from build123d import *

# Parameters (mm, degrees)
F1_DEPTH      = 2.5
F2_SIZE       = 4
F3_SIZE       = 1.99999
F4_R          = 2.49999
F5_R          = 1
F6_DEPTH      = 3.101
F6_DEPTH_BACK = 3.101


# Not quite as in the source:
# - a fillet or chamfer is up to 0.001 mm smaller than in the source, because OpenCascade refuses the exact size


with BuildPart() as f1:
    # F0 (on Top) → F1 (new body, symmetric)
    with BuildSketch(Plane.XY):
        Polygon((-1.1, -50), (0, -50), (1.1, -50), (1.1, -2.5), (3.1, -2.5), (3.1, 50), (1.1, 50), (1.1, 2.5), (0, 2.5), (-1.1, 2.5), (-1.1, 50), (-3.1, 50), (-3.1, -2.5), (-1.1, -2.5), align=None)
    extrude(amount=F1_DEPTH, both=True)

    # F2
    f2_edges = [f1.edges().sort_by_distance(p)[0] for p in [
        (0, -50, -2.5),
    ]]
    chamfer(f2_edges, length=F2_SIZE)

    # F3 (size 2 in the source; OpenCascade refuses exactly that, so slightly less here)
    f3_edges = [f1.edges().sort_by_distance(p)[0] for p in [
        (1.1, -2.5, 0),
        (-1.1, -2.5, 0),
    ]]
    chamfer(f3_edges, length=F3_SIZE)

    # F4 (radius 2.5 in the source; OpenCascade refuses exactly that, so slightly less here)
    f4_edges = [f1.edges().sort_by_distance(p)[0] for p in [
        (2.1, 50, 2.5),
        (-2.1, 50, 2.5),
        (-2.1, 50, -2.5),
        (2.1, 50, -2.5),
        (0, 2.5, -2.5),
        (0, 2.5, 2.5),
    ]]
    fillet(f4_edges, radius=F4_R)

    # F5 (on Right) → F6 (cut, two sides)
    with BuildSketch(Plane.YZ) as f6_sk:
        with Locations((5, 0)):
            Circle(F5_R)
        with Locations((47.5, 0)):
            Circle(F5_R)
    extrude(amount=-F6_DEPTH, mode=Mode.SUBTRACT)
    extrude(f6_sk.sketch, amount=F6_DEPTH_BACK, mode=Mode.SUBTRACT)


solid = f1.part
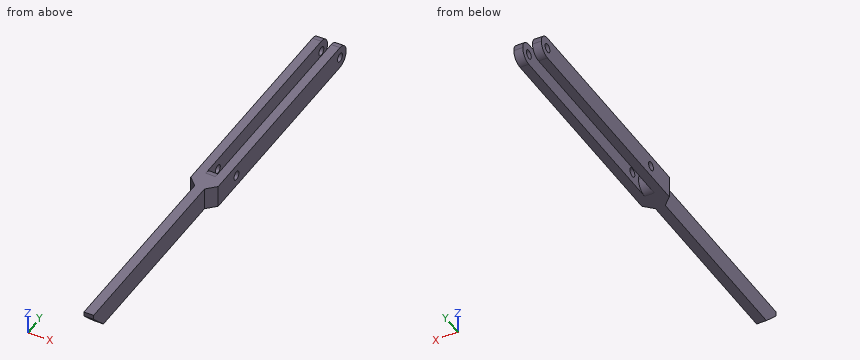
CAD build for the part. Positions are in the model's coordinates, mm. Round coordinates to 2 decimals unless told otherwise and drop trailing zeros. Loops run counter-clockwise (first coordinate to the right, second up) from the corner with the lowest first, then second, coordinate; pieces in that order, holes last.
(1) Cut at B-B (x = 2.25). State how many separate pieces and enclosed holes the cut face has, plus the area to 3 significant figures.
(2) Cut at A-A (y = 5). Give the cut face in (x, z), plus the area to 3 significant figures.
(3) Wall check: line 1 along Y through (x, z) = (2.5, 0); line 2 along X through (y, z) = (17, -0.4); line 3 along Z through (x, y) = (-1.6, 47.5). Give the ranges that are in metal, low to high.
(4) Cut at C-C (y = -39). Give the cut face in (x, z).
Findings below:
1. separate pieces: 1
1. enclosed holes: 2
1. area: 258 mm2
2. outline: (-3.1, -2.5) - (-1.1, -2.5) - (-1.1, -1) - (-3.1, -1) - close; (-3.1, 1) - (-1.1, 1) - (-1.1, 2.5) - (-3.1, 2.5) - close; (1.1, -2.5) - (3.1, -2.5) - (3.1, -1) - (1.1, -1) - close; (1.1, 1) - (3.1, 1) - (3.1, 2.5) - (1.1, 2.5) - close
2. area: 12.0 mm2
3. line 1: y = -3.1 to 4, 6 to 46.5, 48.5 to 50
3. line 2: x = -3.1 to -1.1, 1.1 to 3.1
3. line 3: z = -2.5 to -1, 1 to 2.5
4. outline: (-1.1, -2.5) - (1.1, -2.5) - (1.1, 2.5) - (-1.1, 2.5) - close
